from build123d import *

# Parameters (mm, degrees)
SKETCH_1_R      = 1.65
EXTRUDE_1_DEPTH = 4
CHAMFER_1_SIZE  = 2
CHAMFER_2_SIZE  = 1
CHAMFER_3_SIZE  = 0.4


with BuildPart() as part:
    # 草图1 → 凸台-拉伸1 (new body)
    with BuildSketch(Plane(origin=(0, 0, 0), x_dir=(1, 0, 0), z_dir=(0, 1, 0))):
        with BuildLine():
            Line((2, 0), (16, 0))
            ThreePointArc((16, 0), (17.414213562, 0.585786438), (18, 2))
            Line((18, 2), (18, 10))
            ThreePointArc((18, 10), (17.414213562, 11.414213562), (16, 12))
            Line((16, 12), (2, 12))
            ThreePointArc((2, 12), (0.585786438, 11.414213562), (0, 10))
            Line((0, 10), (0, 2))
            ThreePointArc((0, 2), (0.585786438, 0.585786438), (2, 0))
        make_face()
        with Locations(Location((6, 6, 0), (0, 0, 270))):
            Circle(SKETCH_1_R, mode=Mode.SUBTRACT)
    extrude(amount=EXTRUDE_1_DEPTH)

    # 倒角1
    chamfer_1_edges = [part.edges().sort_by_distance(p)[0] for p in [
        (6, 4, -7.65),
    ]]
    chamfer(chamfer_1_edges, length=CHAMFER_1_SIZE)

    # 倒角2
    chamfer_2_edges = [part.edges().sort_by_distance(p)[0] for p in [
        (0.585786438, 4, -11.414213562),
        (0, 4, -6),
        (0.585786438, 4, -0.585786438),
        (9, 4, 0),
        (17.414213562, 4, -0.585786438),
        (18, 4, -6),
        (17.414213562, 4, -11.414213562),
        (9, 4, -12),
    ]]
    chamfer(chamfer_2_edges, length=CHAMFER_2_SIZE)

    # 倒角3
    chamfer_3_edges = [part.edges().sort_by_distance(p)[0] for p in [
        (0, 0, -6),
        (0.585786438, 0, -11.414213562),
        (9, 0, -12),
        (17.414213562, 0, -11.414213562),
        (18, 0, -6),
        (17.414213562, 0, -0.585786438),
        (9, 0, 0),
        (0.585786438, 0, -0.585786438),
    ]]
    chamfer(chamfer_3_edges, length=CHAMFER_3_SIZE)


solid = part.part
Could you check a few things on this model? Use its own coordinates, in mm. Give positions to 0.01 mm unless a question says otherwise; leave off trailing zeros. Order: outer loops, then holes, each group sorted by start corner. A loop starts at its lowest first (then second) coordinate and runs counter-clockwise, first axis right, second up. Notation, with made-up numbers: (38.5, -28) - (62.5, -28) arc R16 ccw to (62.5, -14) - close; hole circle Ø3 at (-6.75, -30). An arc over 180 degrees is marked (long way). Return JSON: item names as keys, results as strings. Group by question number.
Q1. Suppose I cut it at C-C, the plane y = 2.4. Please give me the cut outline in (x, z), and give its area (3 significant figures).
Q2. Suppose I cut it at A-A, the plane x = 6. Please give me the cut outline in (y, z).
Q3. Suppose I cut it at B-B, the plane z = -6. Please give me the cut outline in (x, y).
Q4. Suppose I cut it at D-D, the plane x = 11.5. Please give me the cut outline in (y, z), and give its area (3 significant figures).
Q5. Please list where these lines run through material, in increasing order: line 1 along X through (y, z) = (0.75, -6); line 2 along Z through (x, y) = (4.75, 0.6); line 3 along Z through (x, y) = (3.75, 3.65). Write a range as [from, to].
Resolved:
{
 "1": {"outline": "(0, -10) arc R2 ccw to (2, -12) - (16, -12) arc R2 ccw to (18, -10) - (18, -2) arc R2 ccw to (16, 0) - (2, 0) arc R2 ccw to (0, -2) - close; hole circle Ø4.1 at (6, -6)", "area": "199 mm2"},
 "2": {"outline": "(0, -11.6) - (0.4, -12) - (3, -12) - (4, -11) - (4, -9.65) - (2, -7.65) - (0, -7.65) - close; (0, -4.35) - (2, -4.35) - (4, -2.35) - (4, -1) - (3, 0) - (0.4, 0) - (0, -0.4) - close"},
 "3": {"outline": "(0, 0.4) - (0.4, 0) - (4.35, 0) - (4.35, 2) - (2.35, 4) - (1, 4) - (0, 3) - close; (7.65, 0) - (17.6, 0) - (18, 0.4) - (18, 3) - (17, 4) - (9.65, 4) - (7.65, 2) - close"},
 "4": {"outline": "(0, -11.6) - (0.4, -12) - (3, -12) - (4, -11) - (4, -1) - (3, 0) - (0.4, 0) - (0, -0.4) - close", "area": "46.8 mm2"},
 "5": {"line 1": "x = [0, 4.35], [7.65, 18]", "line 2": "z = [-12, -7.08], [-4.92, 0]", "line 3": "z = [-11.35, -8.41], [-3.59, -0.65]"}
}
